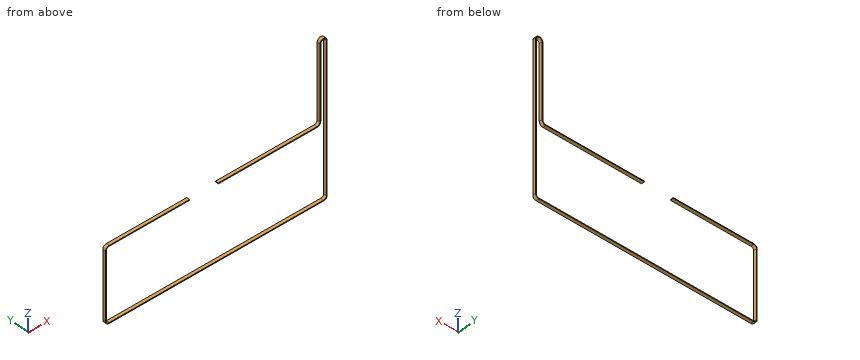
from build123d import *

# Parameters (mm, degrees)
BOSS_EXTRUDE1_DEPTH = 6


with BuildPart() as part:
    # Sketch1 → Boss-Extrude1 (new body)
    with BuildSketch(Plane(origin=(0, 321, 0), x_dir=(1, 0, 0), z_dir=(0, 1, 0))):
        with BuildLine():
            Line((195.6, 23.007337011), (3.974945104, 23.007337011))
            Line((3.974945104, 23.007337011), (3.974945104, 21.507337011))
            Line((3.974945104, 21.507337011), (195.6, 21.507337011))
            ThreePointArc((195.6, 21.507337011), (199.842640687, 19.749977698), (201.6, 15.507337011))
            Line((201.6, 15.507337011), (201.6, -129))
            ThreePointArc((201.6, -129), (208.496418687, -135.899999071), (215.399996282, -129.007162626))
            Line((215.399996282, -129.007162626), (215.699996282, 159.992837374))
            ThreePointArc((215.699996282, 159.992837374), (213.681568504, 164.876503762), (208.8, 166.9))
            Line((208.8, 166.9), (-208.5, 166.9))
            ThreePointArc((-208.5, 166.9), (-213.37903679, 164.87903679), (-215.4, 160))
            Line((-215.4, 160), (-215.4, 28.457337011))
            ThreePointArc((-215.4, 28.457337011), (-213.37903679, 23.578300221), (-208.5, 21.557337011))
            Line((-208.5, 21.557337011), (-52.025054896, 21.557337011))
            Line((-52.025054896, 21.557337011), (-52.025054896, 23.057337011))
            Line((-52.025054896, 23.057337011), (-208.5, 23.057337011))
            ThreePointArc((-208.5, 23.057337011), (-212.318376618, 24.638960392), (-213.9, 28.457337011))
            Line((-213.9, 28.457337011), (-213.9, 160))
            ThreePointArc((-213.9, 160), (-212.318376618, 163.818376618), (-208.5, 165.4))
            Line((-208.5, 165.4), (208.8, 165.4))
            ThreePointArc((208.8, 165.4), (212.62035796, 163.816394249), (214.199997091, 159.994394467))
            Line((214.199997091, 159.994394467), (213.899997091, -129.005605533))
            ThreePointArc((213.899997091, -129.005605533), (208.497197233, -134.399999273), (203.1, -129))
            Line((203.1, -129), (203.1, 15.507337011))
            ThreePointArc((203.1, 15.507337011), (200.903300859, 20.81063787), (195.6, 23.007337011))
        make_face()
    extrude(amount=-BOSS_EXTRUDE1_DEPTH)


solid = part.part
Work out the finished part from the listing and answer in its coordinate system (mm). Give positions to 0.01 mm unless a question says otherwise; leave off trailing zeros. Loops run counter-clockwise (first coordinate to the right, second up) from the corner with the lowest first, then second, coordinate; pieces in that order, holes last. Notation, with made-up numbers: (20.5, -37.75) -> (54.5, -37.75) arc R16 cw to (54.5, -30.75) -> close; hole circle Ø4 at (78.25, 21.5). An arc over 180 degrees is marked (long way). Use a Markdown table: item, result. Add a question column.
1. Flat-ended cylindrical pins translate along their axes: pin 1 Ø1.2 at (y, z) = (317.5, -22.5) entering from +X; pin 2 Ø3 at (y, z) = (315.5, 9) entering from +X; pin 3 Ø1 at (y, z) = (316, 62.5) entering from -X; pin 4 Ø8 at (x, z) = (58.5, -24.5) entering from -Y. Find the tip coordinate at first contact, or state that the pin passes through.
2. Section B-B on y = 319.4 is taken. Determine the outline of the cut face in (x, z), and give its area (3 significant figures).
3. Section C-C on z = 15 is taken. Determine the outline of the cut face in (x, y), and give its area (3 significant figures).
4. Section A-A on x = -149 is taken. Determine the outline of the cut face in (y, z), and give its area (3 significant figures).
5. Find the intervals of material crossed by probe 1 along Z at (x, y) = (131.5, 315.2); probe 2 along X at (y, z) = (316.1, 29.5); probe 3 along X at (y, z) = (318.7, 99), in increasing order.
Results below:
| question | item | result |
|---|---|---|
| 1 | pin 1 | stops at x = 215.56 |
| 1 | pin 2 | stops at x = 215.53 |
| 1 | pin 3 | stops at x = 201.6 |
| 1 | pin 4 | stops at y = 315 |
| 2 | outline | (-215.4, -160) arc R6.9 ccw to (-208.5, -166.9) -> (208.8, -166.9) arc R6.9 ccw to (215.7, -159.99) -> (215.4, 129.01) arc R6.9 ccw to (201.6, 129) -> (201.6, -15.51) arc R6 cw to (195.6, -21.51) -> (3.97, -21.51) -> (3.97, -23.01) -> (195.6, -23.01) arc R7.5 ccw to (203.1, -15.51) -> (203.1, 129) arc R5.4 cw to (213.9, 129.01) -> (214.2, -159.99) arc R5.4 cw to (208.8, -165.4) -> (-208.5, -165.4) arc R5.4 cw to (-213.9, -160) -> (-213.9, -28.46) arc R5.4 cw to (-208.5, -23.06) -> (-52.03, -23.06) -> (-52.03, -21.56) -> (-208.5, -21.56) arc R6.9 ccw to (-215.4, -28.46) -> close |
| 2 | area | 2,080 mm^2 |
| 3 | outline | (201.6, 315) -> (203.1, 315) -> (203.1, 321) -> (201.6, 321) -> close; (214.02, 315) -> (215.52, 315) -> (215.52, 321) -> (214.02, 321) -> close |
| 3 | area | 18.0 mm^2 |
| 4 | outline | (315, -166.9) -> (321, -166.9) -> (321, -165.4) -> (315, -165.4) -> close; (315, -23.06) -> (321, -23.06) -> (321, -21.56) -> (315, -21.56) -> close |
| 4 | area | 18.0 mm^2 |
| 5 | probe 1 | z = -166.9 to -165.4, -23.01 to -21.51 |
| 5 | probe 2 | x = 201.6 to 203.1, 214 to 215.5 |
| 5 | probe 3 | x = 201.6 to 203.1, 213.93 to 215.43 |
